```python
from build123d import *

# Parameters (mm, degrees)
F0_R     = 7.9375
F1_DEPTH = 13.716
F2_R     = 3.175


with BuildPart() as f1:
    # F0 (on Top) → F1 (new body)
    with BuildSketch(Plane.XY):
        Polygon((6.874077, 11.90625), (-6.874077, 11.90625), (-13.748153, 0), (-6.874077, -11.90625), (6.874077, -11.90625), (13.748153, 0), align=None)
        Circle(F0_R, mode=Mode.SUBTRACT)
    extrude(amount=F1_DEPTH)

    # F2
    f2_edges = [f1.edges().sort_by_distance(p)[0] for p in [
        (-13.748153, 0, 6.858),
        (10.311115, -5.953125, 0),
        (13.748153, 0, 6.858),
        (6.874077, -11.90625, 6.858),
        (-6.874077, -11.90625, 6.858),
        (6.874077, 11.90625, 6.858),
        (-6.874077, 11.90625, 6.858),
        (0, -11.90625, 0),
        (-10.311115, -5.953125, 0),
        (-10.311115, 5.953125, 0),
        (0, 11.90625, 0),
        (10.311115, 5.953125, 0),
    ]]
    fillet(f2_edges, radius=F2_R)


solid = f1.part
```
Geometry: final body of the model. Coordinates: model frame, mm. Coordinates: 2 decimals unless noted, no trailing zeros. Order: outer loops, then holes, each group sorted by start corner. A loop starts at its lowest first (then second) coordinate and runs counter-clockwise, first axis right, second up.
Item 1: Draft query along Y for faces 1 (the face through (-1.72, -7.75, 6.76)), 2 (the face through (-6.61, 11.49, 8.52)), 3 (the face through (10.28, -6.01, 8.37)). Return one class per face: released by +Y, released by -Y, zero draft, split by the parting line, or undercut.
Answer:
face 1: undercut
face 2: released by +Y
face 3: released by -Y
Item 2: Section query D-D (x = -2.75). Output: boundary loops of the cut face in (y, z) (3 decimals), then the cut area to 3 significant figures.
Answer:
outline: (-11.906, 3.175) arc R3.175 ccw to (-8.731, 0) - (-7.446, 0) - (-7.446, 13.716) - (-11.906, 13.716) - close; (7.446, 0) - (8.731, 0) arc R3.175 ccw to (11.906, 3.175) - (11.906, 13.716) - (7.446, 13.716) - close
area: 118 mm2
Item 3: Section query C-C (z = 1.25). Output: boundary loops of the cut face in (x, y) (1 decimal), then the cut area to 3 significant figures.
Answer:
outline: (-12.3, -1.3) - (-7.2, -10) arc R2.5 ccw to (-5, -11.3) - (5, -11.3) arc R2.5 ccw to (7.2, -10) - (12.3, -1.3) arc R2.5 ccw to (12.3, 1.3) - (7.2, 10) arc R2.5 ccw to (5, 11.3) - (-5, 11.3) arc R2.5 ccw to (-7.2, 10) - (-12.3, 1.3) arc R2.5 ccw to start; hole circle Ø15.9 at (0, 0)
area: 239 mm2
Item 4: Contact query for flat-ended pins moving along their axis: P1, Ø8, axis at y = 6, z = 4.5, coming from the +X side; P2, Ø4, axis at y = -8.5, z = 1.5, coming from the -X side. Output: stop coordinate, or through.
Answer:
P1: stops at x = 12.59
P2: stops at x = -9.76
Item 5: Material intervals for line 1 along Y through (x, z) = (0, 10.75); line 2 along X through (y, z) = (-3, 2); line 3 along Y through (x, z) = (4.5, 4.25), sorted ascending.
Answer:
line 1: y = -11.91 to -7.94, 7.94 to 11.91
line 2: x = -11.76 to -7.35, 7.35 to 11.76
line 3: y = -11.91 to -6.54, 6.54 to 11.91
